Verification items for the finished model (mm, model axes). Face numbers are marked on the shaded views. Round coordinates to 2 decimals unless told otherwise and drop trailing zeros. Order: outer loops, then holes, each group sorted by start corner. A loop starts at its lowest first (then second) coordinate and runs counter-clockwise, first axis right, second up. Notation, with made-up numbers: (72.25, 65.5) -> (122.25, 65.5) arc R25 ccw to (122.25, 91.5) -> close; hole circle Ø10 at (37.5, -37.75). An arc over 180 degrees is marked (long way). Return JSON: item names as keys, results as strings. Group by question number.
1) Section check B-B on y = 0. Enter the section's corners in (x, z).
2) Section check A-A on x = 0. Enter the section's corners in (y, z), plus the area to 3 significant figures.
3) Section check C-C on z = 2.85. Enter the section's corners in (x, y), plus the area to 3 significant figures.
4) Section check D-D on y = -7.5. Enter the section's corners in (x, z).
5) Scan lines: L1, parallel to Y at x = 0, z = 3.85; L2, parallel to X at y = -7, z = 3.5 (3 decimals); L3, parallel to X at y = -8, z = 1.55. Record each from-to range of solid material in increasing order.
6) Draft check along X on the marked faces 1, 2 and 3. Enter one of: pulls with the +X half, pulls with the -X half, needs draft (parallel to the pull), parting line crosses it, or undercut.
7) Depth check by flat-ended pin: pin 1 (4 mm diameter, centred on x = 0, y = 15, fed in from +Z); pin 2 (1.5 mm diameter, centred on y = -3.5, z = 2, fed in from +X); pin 3 (1.5 mm diameter, centred on y = 3.5, z = 3.5, fed in from -X). Enter the tip coordinate at first touch or a pass-through.
Solid Edge part; units mm, degrees
sketch "Sketch1" plane through (0, 0, 0) normal (0, 0, 1) x (1, 0, 0)
  circle A0 centre (0, 0) radius 10
  circle A1 centre (-12.9904, -7.5) radius 1.5
  circle A2 centre (12.9904, -7.5) radius 1.5
  circle A3 centre (0, 0) radius 20
  circle A4 centre (0, 15) radius 1.5
extrude "Protrusion1" add sketch "Sketch1" along normal blind 5
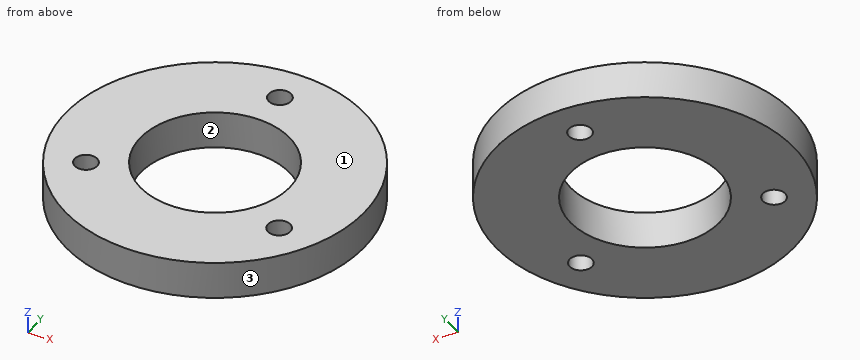
Check result:
{
 "1": {"outline": "(-20, 0) -> (-10, 0) -> (-10, 5) -> (-20, 5) -> close; (10, 0) -> (20, 0) -> (20, 5) -> (10, 5) -> close"},
 "2": {"outline": "(-20, 0) -> (-10, 0) -> (-10, 5) -> (-20, 5) -> close; (10, 0) -> (13.5, 0) -> (13.5, 5) -> (10, 5) -> close; (16.5, 0) -> (20, 0) -> (20, 5) -> (16.5, 5) -> close", "area": "85.0 mm^2"},
 "3": {"outline": "circle Ø40 at (0, 0); hole circle Ø3 at (-12.99, -7.5); hole circle Ø20 at (0, 0); hole circle Ø3 at (0, 15); hole circle Ø3 at (12.99, -7.5)", "area": "921 mm^2"},
 "4": {"outline": "(-18.54, 0) -> (-14.49, 0) -> (-14.49, 5) -> (-18.54, 5) -> close; (-11.49, 0) -> (-6.61, 0) -> (-6.61, 5) -> (-11.49, 5) -> close; (6.61, 0) -> (11.49, 0) -> (11.49, 5) -> (6.61, 5) -> close; (14.49, 0) -> (18.54, 0) -> (18.54, 5) -> (14.49, 5) -> close"},
 "5": {"L1": "-20 to -10, 10 to 13.5, 16.5 to 20", "L2": "-18.735 to -14.405, -11.576 to -7.141, 7.141 to 11.576, 14.405 to 18.735", "L3": "-18.33 to -14.4, -11.58 to -6, 6 to 11.58, 14.4 to 18.33"},
 "6": {"face 1": "needs draft", "face 2": "undercut", "face 3": "parting line crosses it"},
 "7": {"pin 1": "z = 5", "pin 2": "x = 19.81", "pin 3": "x = -19.81"}
}
